from build123d import *

# Parameters (mm, degrees)
BOSS_EXTRUDE1_DEPTH = 9
SKETCH2_R           = 1.585
CUT_EXTRUDE1_DEPTH  = 32
SKETCH3_W           = 8
SKETCH3_H           = 3
CUT_EXTRUDE4_DEPTH  = 32


with BuildPart() as part:
    # Sketch1 → Boss-Extrude1 (new body)
    with BuildSketch(Plane(origin=(0, 0, 0), x_dir=(1, 0, 0), z_dir=(0, 1, 0))):
        with BuildLine():
            Line((25.334549447, 26.26861883), (39.718507893, 26.26861883))
            ThreePointArc((39.718507893, 26.26861883), (43.74975272, 21.687555144), (47.780997547, 26.26861883))
            Line((47.780997547, 26.26861883), (62.176678451, 26.26861883))
            ThreePointArc((62.176678451, 26.26861883), (43.755613949, 9.05519235), (25.334549447, 26.26861883))
        make_face()
    extrude(amount=BOSS_EXTRUDE1_DEPTH)

    # Sketch2 → Cut-Extrude1 (cut)
    with BuildSketch(Plane(origin=(43.755613949, 0.001959277, -52.26861883), x_dir=(1, 0, 0), z_dir=(0, 0, 1))):
        with Locations((9.500000009, 4.5)):
            Circle(SKETCH2_R)
        with Locations((-9.499999996, 4.5)):
            Circle(SKETCH2_R)
    extrude(amount=CUT_EXTRUDE1_DEPTH, mode=Mode.SUBTRACT)

    # Sketch3 → Cut-Extrude4 (cut)
    with BuildSketch(Plane(origin=(0, 9, 0), x_dir=(1, 0, 0), z_dir=(0, 1, 0))):
        with Locations((52.74975272, 21.76861883)):
            Rectangle(SKETCH3_W, SKETCH3_H)
        with Locations((34.74975272, 21.76861883)):
            Rectangle(SKETCH3_W, SKETCH3_H)
    extrude(amount=-CUT_EXTRUDE4_DEPTH, mode=Mode.SUBTRACT)


solid = part.part
Could you check a few things on this model? Use its own coordinates, in mm. A direction names the side the tool comes from. Round coordinates to 2 decimals unless told otherwise and drop trailing zeros. Order: outer loops, then holes, each group sorted by start corner. A loop starts at its lowest first (then second) coordinate and runs counter-clockwise, first axis right, second up. Notation, with made-up numbers: M 59.25,89.25 L 65.25,89.25 A14 cw 65.25,102.25 Z; hole C -27.75,48.5 d8. An arc over 180 degrees is marked long. One line per item, written item: value.
(1) Imagine slicing it at C-C (x = 35). Write out the boundary of the cut face in (y, z), and give its area (3 significant figures).
Ans:
outline: M 0,-26.27 L 3.1,-26.27 L 3.1,-23.27 L 0,-23.27 Z; M 0,-20.27 L 9,-20.27 L 9,-11.26 L 0,-11.26 Z; M 5.9,-26.27 L 9,-26.27 L 9,-23.27 L 5.9,-23.27 Z
area: 99.7 mm^2
(2) I'm going to push flat-ended pins straight in: P1, Ø1.5, axis at y = 5.5, z = -22, coming from the -X side; P2, Ø3.5, axis at y = 3.5, z = -22.5, coming from the +X side; P3, Ø1.5, axis at y = 7, z = -17, coming from the +X side; P4, Ø5, axis at x = 34, z = -19, coming from the -Y side. Where does each tip first touch, or does it pass through?
Ans:
P1: stops at x = 25.92
P2: stops at x = 61.93
P3: stops at x = 59.42
P4: stops at y = 0
(3) I need wall thicknesses on line 1 along Z through (x, y) = (31.5, 2.25); line 2 along Z through (x, y) = (53, 2); line 3 along X through (y, z) = (3.5, -24). Which ranges of each line are inside material? Lowest first, please. Write a range as from..to.
Ans:
line 1: z = -26.27..-23.27, -20.27..-13.71
line 2: z = -26.27..-23.27, -20.27..-11.54
line 3: x = 25.63..33.03, 35.48..40.08, 47.42..52.03, 54.48..61.88
(4) Which directions (+Z, -Z, +X, -X, +Y, -Y) give clear straight access to the entire face, cutting with the end or side of a thin tool? Please do faces 4 (the flat face through (52, 6, -23.269)), 5 (the flat face through (32, 4, -26.269)), 6 (the cylindrical face through (54.72, 3.895, -24.79)).
Ans:
face 4: +Y, -Y
face 5: -Z, +X, -X, +Y, -Y
face 6: -Z
(5) If we mould it in two halves opening along Y, with no side actions, what happens to faces 1 (the flat face through (44, 9, -18)), 2 (the flat face through (55, 4, -26.269)), 3 (the cylindrical face through (32.672, 4.572, -24.79))? For each: released by +Y, released by -Y, zero draft, split by the parting line, or undercut.
Ans:
face 1: released by +Y
face 2: zero draft
face 3: undercut
(6) Imagine slicing it at D-D (z = -21.25). Write out the boundary of the cut face in (x, y).
Ans:
outline: M 26.39,0 L 30.75,0 L 30.75,9 L 26.39,9 Z; M 38.75,0 L 48.75,0 L 48.75,9 L 38.75,9 Z; M 56.75,0 L 61.12,0 L 61.12,9 L 56.75,9 Z
(7) Imagine slicing it at B-B (z = -24.75). Write out the boundary of the cut face in (x, y) (3 decimals), and give its area (3 significant figures).
Ans:
outline: M 25.501,0 L 39.811,0 L 39.811,9 L 25.501,9 Z; M 47.689,0 L 62.01,0 L 62.01,9 L 47.689,9 Z; hole C 34.256,4.502 d3.17; hole C 53.256,4.502 d3.17
area: 242 mm^2
